Print and shaded views of the part. All mm, measured from the part's lowest x, y and z. Round coordinates to 2 decimals unless told otherwise and drop trailing zeros. Write each loop counter-clockwise with the first axis right and the second up, starting at its lowest first coordinate (ties: lowest second). Pieces come first, ordered by that corner, then holes. Notation, with made-up numbers: (30, -33) - (54, -33) arc R19 ccw to (54, -7) - close; hole circle Ø4 at (87, 67.5). An arc over 180 degrees is marked (long way). One line per item, written item: value.
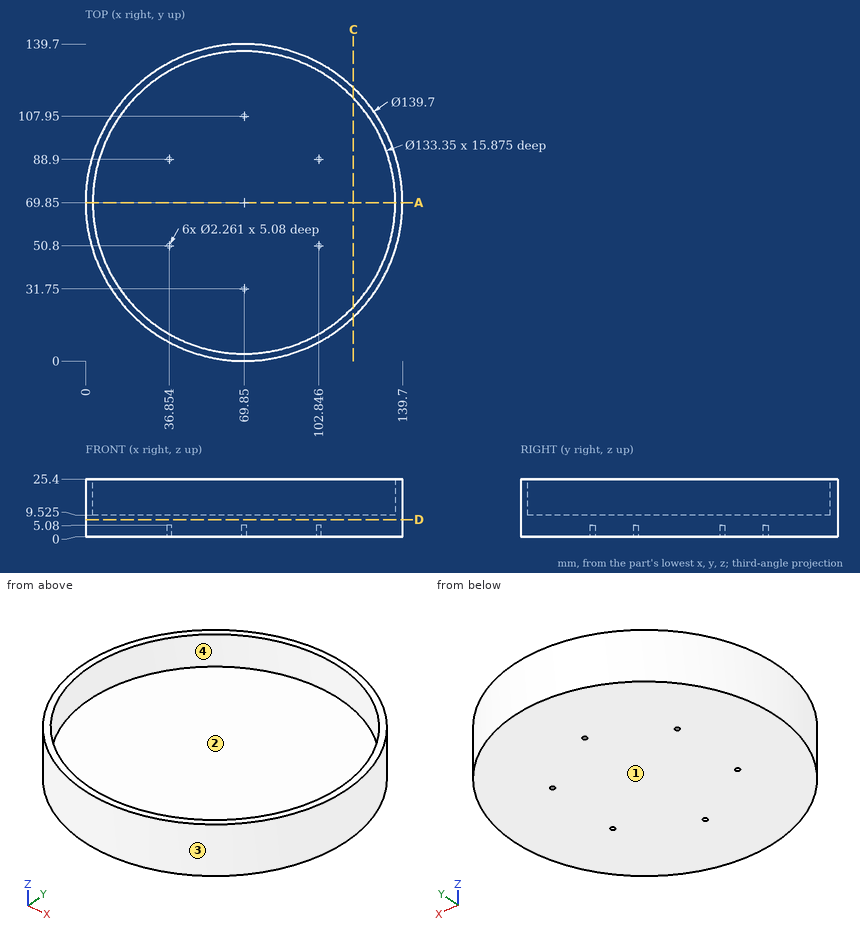
1. Wall check: probe 1 along Y at (x, z) = (69.85, 4.15); probe 2 along X at (y, z) = (88.9, 1.5) (1 decimal); probe 3 along Z at (x, y) = (68, 82.5) (1 decimal). Give the ranges that are in metal, low to high. Write a range as [from, to].
Report:
probe 1: [0, 30.62], [32.88, 106.82], [109.08, 139.7]
probe 2: [2.6, 35.7], [38, 101.7], [104, 137.1]
probe 3: [0, 9.5]
2. Band-saw the part on C-C on x = 118. Write the cut outline in (y, z) (1 decimal).
Report:
outline: (19.2, 0) - (120.5, 0) - (120.5, 25.4) - (116, 25.4) - (116, 9.5) - (23.7, 9.5) - (23.7, 25.4) - (19.2, 25.4) - close
3. Band-saw the part on D-D on z = 7.5. Write the cut outline in (x, y).
Report:
outline: circle Ø139.7 at (69.85, 69.85)
4. Drop flat-ended pins along their axis: pin 1 (2 mm diameter, centred on x = 102.85, y = 88.9, fed in from +Z) (3 decimals); pin 2 (1.1 mm diameter, centred on x = 102.5, y = 50.5, fed in from -Z); pin 3 (6 mm diameter, centred on x = 69.5, z = 4.5, fed in from -Y). Give the stop position or say it passes through.
Report:
pin 1: z = 9.525
pin 2: z = 5.08
pin 3: y = 0
5. Band-saw the part on A-A on y = 69.85. Write the cut outline in (x, z) (1 decimal), plus the area to 3 significant figures.
Report:
outline: (0, 0) - (139.7, 0) - (139.7, 25.4) - (136.5, 25.4) - (136.5, 9.5) - (3.2, 9.5) - (3.2, 25.4) - (0, 25.4) - close
area: 1,430 mm²
6. Mould opens along X. For the marked faces 1, 2, 3 and 4 say: released by +X, released by -X, zero draft, split by the parting line, or undercut.
Report:
face 1: zero draft
face 2: undercut
face 3: split by the parting line
face 4: undercut
